from build123d import *

# Parameters (mm, degrees)
F0_R        = 18
F0_R_2      = 3.5
F1_DEPTH    = 12
F0_R_3      = 1.5
F2_DEPTH    = 16.5
F2_FACE_R   = 3.5
F2_FACE_R_2 = 1.5
F3_DEPTH    = 21
F4_R        = 2.51997
F5_DEPTH    = 1


with BuildPart() as f1:
    # F0 (on Front) → F1 (new body)
    with BuildSketch(Plane.XZ):
        Circle(F0_R)
        Circle(F0_R_2, mode=Mode.SUBTRACT)
    extrude(amount=F1_DEPTH)

    # F0 (on Front) → F2 (join)
    with BuildSketch(Plane.XZ):
        Circle(F0_R_2)
        Circle(F0_R_3, mode=Mode.SUBTRACT)
    extrude(amount=F2_DEPTH)

    # F2_face (on face) → F3 (join)
    with BuildSketch(Plane.XZ.offset(16.5)):
        Circle(F2_FACE_R)
        Circle(F2_FACE_R_2, mode=Mode.SUBTRACT)
    extrude(amount=-F3_DEPTH)

    # F4 (on face) → F5 (join)
    with BuildSketch(Plane.XZ.offset(16.5)):
        Circle(F4_R)
    extrude(amount=-F5_DEPTH)


solid = f1.part
Verification items for the finished model (mm, model axes). A direction names the side the tool comes from. Coordinates: 2 decimals unless noted, no trailing zeros. Order: outer loops, then holes, each group sorted by start corner. A loop starts at its lowest first (then second) coordinate and runs counter-clockwise, first axis right, second up. Notation, with made-up numbers: M 76,-5 L 116,-5 A18 ccw 116,11 Z; hole C 50.25,57.5 d5. An arc over 180 degrees is marked long. One line per item, written item: value. Start each with the question number.
Item 1: Mould release check, pull along X, two halves, no side actions. Record for faces 1 (the cylindrical face through (-1.5, -5.64, 0.07)), 2 (the cylindrical face through (3.233, 2.218, -1.341)), 3 (the flat face through (0, 0, -4)): pulls with the +X half, pulls with the -X half, needs draft (parallel to the pull), parting line crosses it, or undercut.
Item 2: Sectioned sample at D-D on y = -13. Record the cut outline in (x, z), then the cut area to 3 significant figures.
Item 3: Thickness scan on probe 1 along Z at (x, y) = (0, -1.5); probe 2 along Y at (x, z) = (-10, 8.5); probe 3 along Z at (x, y) = (0.5, -0.25). Record the ranges inside material, lowest first.
Item 4: Depth check by flat-ended pin: P1, Ø1.5, axis at y = -12.5, z = -1, coming from the -X side; P2, Ø4, axis at x = -6.5, y = 1, coming from the +Z side; P3, Ø2, axis at y = -5, z = 14, coming from the +X side. Enter the tip coordinate at first touch or a pass-through.
Item 5: Sectioned sample at B-B on x = 0. Record the cut outline in (y, z).
Item 6: Sectioned sample at C-C on y = -9.5. Record the cut outline in (x, z), then the cut area to 3 significant figures.
Item 7: Sectioned sample at A-A on z = 0. Record the cut outline in (x, y).
Item 8: Access from +Z, -Z, +X, -X, +Y, -Y to the whole of each face (thin tool, end or side, straight path). Record for faces 4 (the flat face through (0, -15.5, 0)), 5 (the cylindrical face through (3.233, -14.218, -1.341)), 6 (the flat face through (0, -16.5, 0)).
Calculated:
1. face 1: undercut
1. face 2: parting line crosses it
1. face 3: needs draft
2. outline: C 0,0 d7; hole C 0,0 d3
2. area: 31.4 mm^2
3. probe 1: -18 to -1.5, 1.5 to 18
3. probe 2: -12 to 0
3. probe 3: -17.99 to -1.41, 1.41 to 17.99
4. P1: x = -17.99
4. P2: z = 17.36
4. P3: x = 12.45
5. outline: M -16.5,-3.5 L -12,-3.5 L -12,-18 L 0,-18 L 0,-3.5 L 4.5,-3.5 L 4.5,-1.5 L -15.5,-1.5 L -15.5,1.5 L 4.5,1.5 L 4.5,3.5 L 0,3.5 L 0,18 L -12,18 L -12,3.5 L -16.5,3.5 Z
6. outline: C 0,0 d36; hole C 0,0 d3
6. area: 1,010 mm^2
7. outline: M -18,-12 L -3.5,-12 L -3.5,-16.5 L 3.5,-16.5 L 3.5,-12 L 18,-12 L 18,0 L 3.5,0 L 3.5,4.5 L 1.5,4.5 L 1.5,-15.5 L -1.5,-15.5 L -1.5,4.5 L -3.5,4.5 L -3.5,0 L -18,0 Z
8. face 4: +Y
8. face 5: -Y
8. face 6: +Z, -Z, +X, -X, -Y
